Here's how the part is built. I have some questions about the finished solid (model axes, mm). Face numbers are marked on the shaded views. A direction names the side the tool comes from. Round coordinates to 2 decimals unless told otherwise and drop trailing zeros. Order: outer loops, then holes, each group sorted by start corner. A loop starts at its lowest first (then second) coordinate and runs counter-clockwise, first axis right, second up.
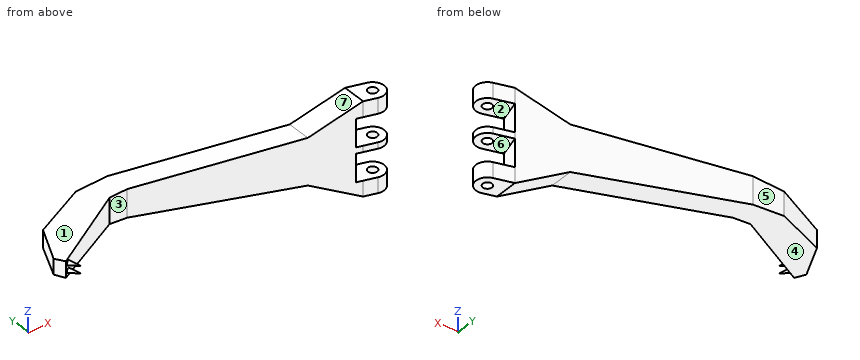
```python
from build123d import *

# Parameters (mm, degrees)
BOSS_EXTRUDE2_DEPTH      = 15
BOSS_EXTRUDE2_DEPTH_BACK = 15
SKETCH3_R                = 1.5
CUT_EXTRUDE2_DEPTH       = 106.264714703
CUT_EXTRUDE2_DEPTH_BACK  = 106.264714703
SKETCH12_OUTSIDE_W       = 130.034
SKETCH12_OUTSIDE_H       = 54.552
BOSS_EXTRUDE3_DEPTH      = 15
BOSS_EXTRUDE3_DEPTH_BACK = 15
SKETCH13_R               = 1.5
CUT_EXTRUDE8_REACH       = 107.495
SKETCH16_W               = 6.181190374
SKETCH16_H               = 9
SKETCH16_W_2             = 3.75


with BuildPart() as part:
    # Sketch3 → Boss-Extrude2 (new, two sides: drawn at the far end of the back side and taken through both)
    with BuildSketch(Plane.XY.offset(-BOSS_EXTRUDE2_DEPTH_BACK)):
        with BuildLine():
            Line((0.970571419, 3.622221849), (-69.482255776, 22.5))
            Line((-69.482255776, 22.5), (-79.701126542, 22.5))
            Line((-79.701126542, 22.5), (-96.234008051, 14.790590741))
            Line((-96.234008051, 14.790590741), (-101.732050808, 3))
            Line((-101.732050808, 3), (-100, 0))
            Line((-100, 0), (-74.714962449, 14.598323237))
            Line((-74.714962449, 14.598323237), (-68.970571419, 14.598323237))
            Line((-68.970571419, 14.598323237), (-0.970571419, -3.622221849))
            ThreePointArc((-0.970571419, -3.622221849), (3.622221849, -0.970571419), (0.970571419, 3.622221849))
        make_face()
        Circle(SKETCH3_R, mode=Mode.SUBTRACT)
    extrude(amount=BOSS_EXTRUDE2_DEPTH + BOSS_EXTRUDE2_DEPTH_BACK)

    # Sketch12 outside → Cut-Extrude2 (cut, two sides: drawn at the far end of the back side and taken through both)
    with BuildSketch(Plane(origin=(0, 0, 0), x_dir=(1, 0, 0), z_dir=(0, 1, 0)).offset(-CUT_EXTRUDE2_DEPTH_BACK)):
        with Locations((-48.991, 0)):
            Rectangle(SKETCH12_OUTSIDE_W, SKETCH12_OUTSIDE_H)
        Polygon((-101.732050808, 2.5), (-101.732050808, -2.5), (-20, -7.5), (-5, -15), (-5, 15), (-20, 7.5), align=None, mode=Mode.SUBTRACT)
    extrude(amount=CUT_EXTRUDE2_DEPTH + CUT_EXTRUDE2_DEPTH_BACK, mode=Mode.SUBTRACT)

    # Sketch13 → Boss-Extrude3 (add, two sides: drawn at the far end of the back side and taken through both)
    with BuildSketch(Plane.XY.offset(-BOSS_EXTRUDE3_DEPTH_BACK)):
        with BuildLine():
            Line((-5, 5.222031639), (-5, -2.542539714))
            Line((-5, -2.542539714), (-0.970571419, -3.622221849))
            ThreePointArc((-0.970571419, -3.622221849), (3.622221849, -0.970571419), (0.970571419, 3.622221849))
            Line((0.970571419, 3.622221849), (-5, 5.222031639))
        make_face()
        Circle(SKETCH13_R, mode=Mode.SUBTRACT)
    extrude(amount=BOSS_EXTRUDE3_DEPTH + BOSS_EXTRUDE3_DEPTH_BACK)

    # Cut-Extrude8: up to this face of the body (flat: up to its plane)
    cut_extrude8_end = Plane(part.part.faces().sort_by_distance((-27.959079365, 3.60932706, 0))[0])
    # Sketch16 → Cut-Extrude8 (cut, up to the picked face)
    with BuildSketch(Plane(origin=(0.970571419, 3.622221849, 0), x_dir=(0.9659258262890683, -0.2588190451025211, 0), z_dir=(0.2588190451025211, 0.9659258262890683, 0)), mode=Mode.PRIVATE) as cut_extrude8_sk1:
        with Locations((-3.090595187, 5.5)):
            Rectangle(SKETCH16_W, SKETCH16_H)
    cut_extrude8_tool1 = split(extrude(cut_extrude8_sk1.sketch, amount=-CUT_EXTRUDE8_REACH, mode=Mode.PRIVATE), bisect_by=cut_extrude8_end, keep=Keep.BOTH, mode=Mode.PRIVATE)
    # Sketch16 → Cut-Extrude8 (cut, up to the picked face)
    with BuildSketch(Plane(origin=(0.970571419, 3.622221849, 0), x_dir=(0.9659258262890683, -0.2588190451025211, 0), z_dir=(0.2588190451025211, 0.9659258262890683, 0)), mode=Mode.PRIVATE) as cut_extrude8_sk2:
        with Locations((-3.090595187, -5.5)):
            Rectangle(SKETCH16_W, SKETCH16_H)
    cut_extrude8_tool2 = split(extrude(cut_extrude8_sk2.sketch, amount=-CUT_EXTRUDE8_REACH, mode=Mode.PRIVATE), bisect_by=cut_extrude8_end, keep=Keep.BOTH, mode=Mode.PRIVATE)
    # Sketch16 → Cut-Extrude8 (cut, up to the picked face)
    with BuildSketch(Plane(origin=(0.970571419, 3.622221849, 0), x_dir=(0.9659258262890683, -0.2588190451025211, 0), z_dir=(0.2588190451025211, 0.9659258262890683, 0)), mode=Mode.PRIVATE) as cut_extrude8_sk3:
        with Locations((1.875, -5.5)):
            Rectangle(SKETCH16_W_2, SKETCH16_H)
    cut_extrude8_tool3 = split(extrude(cut_extrude8_sk3.sketch, amount=-CUT_EXTRUDE8_REACH, mode=Mode.PRIVATE), bisect_by=cut_extrude8_end, keep=Keep.BOTH, mode=Mode.PRIVATE)
    # Sketch16 → Cut-Extrude8 (cut, up to the picked face)
    with BuildSketch(Plane(origin=(0.970571419, 3.622221849, 0), x_dir=(0.9659258262890683, -0.2588190451025211, 0), z_dir=(0.2588190451025211, 0.9659258262890683, 0)), mode=Mode.PRIVATE) as cut_extrude8_sk4:
        with Locations((1.875, 5.5)):
            Rectangle(SKETCH16_W_2, SKETCH16_H)
    cut_extrude8_tool4 = split(extrude(cut_extrude8_sk4.sketch, amount=-CUT_EXTRUDE8_REACH, mode=Mode.PRIVATE), bisect_by=cut_extrude8_end, keep=Keep.BOTH, mode=Mode.PRIVATE)
    add(cut_extrude8_tool1.solids().sort_by(Axis((-2.014714, 4.422127, -5.5), (-0.2588190451025211, -0.9659258262890683, 0)))[0], mode=Mode.SUBTRACT)
    add(cut_extrude8_tool2.solids().sort_by(Axis((-2.014714, 4.422127, 5.5), (-0.2588190451025211, -0.9659258262890683, 0)))[0], mode=Mode.SUBTRACT)
    add(cut_extrude8_tool3.solids().sort_by(Axis((2.781682, 3.136936, 5.5), (-0.2588190451025211, -0.9659258262890683, 0)))[0], mode=Mode.SUBTRACT)
    add(cut_extrude8_tool4.solids().sort_by(Axis((2.781682, 3.136936, -5.5), (-0.2588190451025211, -0.9659258262890683, 0)))[0], mode=Mode.SUBTRACT)

    # Boss-Extrude4 cone 1 section (through the dimple's axis) → Boss-Extrude4 (revolve)
    with BuildSketch(Plane(origin=(-98.700961894, 0.75, 1.183324765), x_dir=(0, 0, 1), z_dir=(0.866025404, 0.5, 0))):
        Polygon((0, 0), (0.75, 0), (0, 3.528472582), align=None)
    revolve(axis=Axis((-98.700961894, 0.75, 1.183324765), (0.5, -0.866025404, 0)))

    # Boss-Extrude4 cone 2 section (through the dimple's axis) → Boss-Extrude4 cone 2 (revolve)
    with BuildSketch(Plane(origin=(-98.700961894, 0.75, -1.183324765), x_dir=(0, 0, 1), z_dir=(0.866025404, 0.5, 0))):
        Polygon((0, 0), (0.75, 0), (0, 3.528472582), align=None)
    revolve(axis=Axis((-98.700961894, 0.75, -1.183324765), (0.5, -0.866025404, 0)))


solid = part.part
```
1. If we section it at C-C, the plane y = 17.5: Write out the boundary of the cut face in (x, z), and give its area (3 significant figures).
Evaluation:
outline: (-90.42, -3.19) - (-50.82, -5.61) - (-50.82, 5.61) - (-90.42, 3.19) - close
area: 349 mm2
2. If we section it at A-A, the plane x = -3.5: Write out the boundary of the cut face in (y, z).
Evaluation:
outline: (-2.94, -15) - (4.82, -15) - (4.82, -10) - (-2.94, -10) - close; (-2.94, -1) - (4.82, -1) - (4.82, 1) - (-2.94, 1) - close; (-2.94, 10) - (4.82, 10) - (4.82, 15) - (-2.94, 15) - close
3. I need wall thicknesses on probe 1 along X at (y, z) = (0, -13.3); probe 2 along Z at (x, y) = (-81, 14.5); probe 3 along Y at (x, z) = (0, 13.15). Which ranges of each line are inside material? Lowest first, please.
Evaluation:
probe 1: x = -8.4 to -1.5, 1.5 to 3.75
probe 2: z = -3.77 to 3.77
probe 3: y = -3.75 to -1.5, 1.5 to 3.88
4. I'm going to push flat-ended pins straight in: P1, Ø10, axis at y = 18.5, z = 11.5, coming from the +X side; P2, Ø1, axis at x = -21.5, z = 4, coming from the +Y side; P3, Ø1.7, axis at x = -71.5, z = -1.5, coming from the -Y side; P4, Ø1.5, axis at x = -57.5, z = 2.5, coming from the +Y side. Where does each tip first touch, or does it pass through?
Evaluation:
P1: passes through
P2: stops at y = 9.78
P3: stops at y = 14.6
P4: stops at y = 19.49
5. If we mould it in two halves opening along Z, with no side actions, what happens to the marked faces 4, 5, 6 and 7? For each: released by +Z, released by -Z, zero draft, split by the parting line, or undercut.
Evaluation:
face 4: released by -Z
face 5: zero draft
face 6: undercut
face 7: released by +Z
6. On a 3-axis mill with a long thin cutter (end or side, diameter ignored), from which of +Z, -Z, +X, -X, +Y, -Y can I reach the whole of each face in a straight line? I mean the marked faces 1, 2 and 3. Say none if no direction works.
Evaluation:
face 1: +Z, -X, +Y, -Y
face 2: +X, -Y
face 3: +Z, -Z, -Y
7. If we section it at B-B, the plane x = -71.5: Write out the boundary of the cut face in (y, z).
Evaluation:
outline: (14.6, -4.35) - (22.5, -4.35) - (22.5, 4.35) - (14.6, 4.35) - close
